For this review, take the finished solid that the model builds, in its own axes (mm). Face numbers are marked on the shaded views. A direction names the side the tool comes from. Give positions to 0.01 mm unless a question says otherwise; leave off trailing zeros. Write each loop counter-clockwise with the first axis right and the second up, starting at its lowest first coordinate (ties: lowest second). Pieces come first, ordered by that corner, then holes. Notation, with made-up numbers: (28, -30.5) -> (54, -30.5) arc R29 ccw to (54, -7.5) -> close; hole circle Ø4 at (-23.75, 72.25). An arc over 180 degrees is marked (long way). Return JSON: item names as keys, results as strings.
from build123d import *

# Parameters (mm, degrees)
SKETCH1_R           = 16.175
SKETCH1_R_2         = 12.4
BOSS_EXTRUDE1_DEPTH = 2
SKETCH1_3_R         = 16.175
SKETCH1_3_R_2       = 12.4
BOSS_EXTRUDE2_DEPTH = 20
SKETCH2_R           = 2.1
CUT_EXTRUDE1_DEPTH  = 39.029218482
CIRPATTERN1_COUNT   = 6


with BuildPart() as part:
    # Sketch1 → Boss-Extrude1 (new body)
    # profile 1 of 3: a face of its own
    with BuildSketch(Plane(origin=(0, 0, 0), x_dir=(1, 0, 0), z_dir=(0, 1, 0))):
        Polygon((-12.22539195, -21.175), (12.22539195, -21.175), (24.4507839, 0), (12.22539195, 21.175), (-12.22539195, 21.175), (-24.4507839, 0), align=None)
        Circle(SKETCH1_R, mode=Mode.SUBTRACT)
    # profile 2 of 3: a face of its own
    with BuildSketch(Plane(origin=(0, 0, 0), x_dir=(1, 0, 0), z_dir=(0, 1, 0))):
        Circle(SKETCH1_R)
        Circle(SKETCH1_R_2, mode=Mode.SUBTRACT)
    # profile 3 of 3: a face of its own
    with BuildSketch(Plane(origin=(0, 0, 0), x_dir=(1, 0, 0), z_dir=(0, 1, 0))):
        Circle(SKETCH1_R_2)
    extrude(amount=-BOSS_EXTRUDE1_DEPTH)

    # Sketch1_3 → Boss-Extrude2 (add)
    # profile 1 of 2: a face of its own
    with BuildSketch(Plane(origin=(0, 0, 0), x_dir=(1, 0, 0), z_dir=(0, 1, 0))):
        Polygon((-12.22539195, -21.175), (12.22539195, -21.175), (24.4507839, 0), (12.22539195, 21.175), (-12.22539195, 21.175), (-24.4507839, 0), align=None)
        with Locations(Location((0, 0, 0), (0, 0, 270))):
            Circle(SKETCH1_3_R, mode=Mode.SUBTRACT)
    # profile 2 of 2: a face of its own
    with BuildSketch(Plane(origin=(0, 0, 0), x_dir=(1, 0, 0), z_dir=(0, 1, 0))):
        with Locations(Location((0, 0, 0), (0, 0, 270))):
            Circle(SKETCH1_3_R_2)
    extrude(amount=BOSS_EXTRUDE2_DEPTH)

    # Sketch2 → Cut-Extrude1 (cut, through all)
    with BuildSketch(Plane.XY):
        with Locations((0, 4.5)):
            Circle(SKETCH2_R)
    cut_extrude1 = extrude(amount=-CUT_EXTRUDE1_DEPTH, mode=Mode.SUBTRACT)

    # CirPattern1: Cut-Extrude1 ×6 about axis
    cirpattern1_axis = Axis((0, 20, 0), (0, -1, 0))
    for i in range(1, CIRPATTERN1_COUNT):
        add(cut_extrude1.rotate(cirpattern1_axis, i * 360 / CIRPATTERN1_COUNT), mode=Mode.SUBTRACT)


solid = part.part
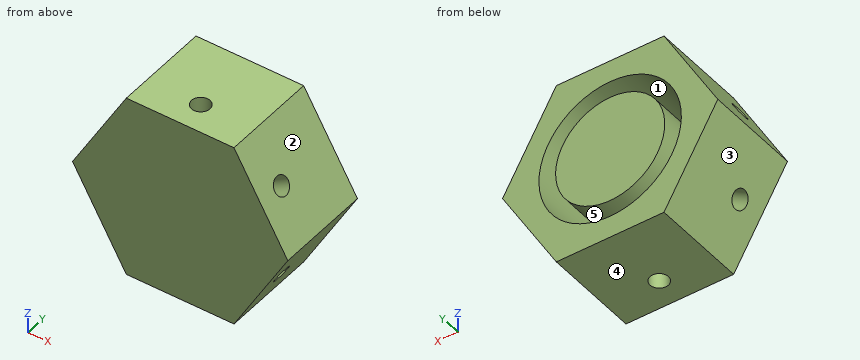
1. To check wall thickness, follow probe 1 along Z at (x, y) = (0, 14) (3 decimals); probe 2 along Z at (x, y) = (17, 4); probe 3 along Y at (x, z) = (0, 6). State the ranges of each line that lie inside material, in increasing order.
Results found:
{"probe 1": "z = -21.175 to -16.175, -12.4 to 12.4, 16.175 to 21.175", "probe 2": "z = -12.91 to -12.17, -7.46 to 7.46, 12.17 to 12.91", "probe 3": "y = -2 to 2.4, 6.6 to 20"}
2. For pin 1 (4 mm diameter, centred on y = 17, z = -16.5, fed in from -X); pin 2 (4 mm diameter, centred on x = 0, y = 4.5, fed in from -Z); pin 3 (1.5 mm diameter, centred on y = 10, z = -11, fed in from +X); pin 4 (3 mm diameter, centred on y = 4, z = 6.5, fed in from +X), all flat-tipped, find the tip position at first contact; note any pin that passes through.
Results found:
{"pin 1": "stops at x = -16.08", "pin 2": "passes through", "pin 3": "stops at x = 18.53", "pin 4": "stops at x = 21.56"}
3. Add section B-B, the plane z = 17.5. State the section outline as (x, y) points, plus the area to 3 significant figures.
Results found:
{"outline": "(-14.35, -2) -> (14.35, -2) -> (14.35, 20) -> (-14.35, 20) -> close; hole circle Ø4.2 at (0, 4.5)", "area": "617 mm²"}
4. Add section C-C, the plane x = 1.5. Count the separate pieces of the cut face and the enclosed holes in it, plus the area to 3 significant figures.
Results found:
{"separate pieces": "4", "enclosed holes": "0", "area": "673 mm²"}
5. Add section A-A, the plane y = 14. State the section outline as (x, z) points (3 decimals).
Results found:
{"outline": "(-24.451, 0) -> (-12.225, -21.175) -> (12.225, -21.175) -> (24.451, 0) -> (12.225, 21.175) -> (-12.225, 21.175) -> close; circle Ø24.8 at (0, 0); hole circle Ø32.35 at (0, 0)"}
6. The part is to be moulded in two halves that separate along X. For the marked faces 3, 4 and 5, say which applies: +X half, -X half, draft (parallel to the pull), parting line (faces both ways), or undercut.
Results found:
{"face 3": "-X half", "face 4": "draft", "face 5": "undercut"}
7. For the marked faces 1 and 2, list the 3-axis set-ups (+Z, -Z, +X, -X, +Y, -Y) from which the entire face can be reached by the end or side of a thin tool; tool diameter is ignored.
Results found:
{"face 1": "+Y", "face 2": "+Z, +X, +Y, -Y"}
8. Add section D-D, the plane x = 21.5. State the section outline as (y, z) points.
Results found:
{"outline": "(-2, -5.11) -> (20, -5.11) -> (20, 5.11) -> (-2, 5.11) -> close"}
